```python
from build123d import *

# Parameters (mm, degrees)
SKETCH_1_R      = 4
EXTRUDE_1_DEPTH = 5


with BuildPart() as part:
    # 草图1 → 凸台-拉伸1 (new body)
    with BuildSketch(Plane.XY):
        with BuildLine():
            Line((-7.924938012, 37.574342627), (-22.446516876, 37.574342627))
            Line((-22.446516876, 37.574342627), (-22.446516876, 34.574342627))
            Line((-22.446516876, 34.574342627), (-13.144515754, 34.574342627))
            Line((-13.144515754, 34.574342627), (-13.144515754, 29.574342627))
            Line((-13.144515754, 29.574342627), (-16.675920201, 29.574342627))
            Line((-16.675920201, 29.574342627), (-16.675920201, 3.864736877))
            ThreePointArc((-16.675920201, 3.864736877), (-13.746988013, -3.206330935), (-6.675920201, -6.135263123))
            Line((-6.675920201, -6.135263123), (4.313762442, -6.135263123))
            ThreePointArc((4.313762442, -6.135263123), (7.499853762, 0.046835335), (4.2368016, 6.188659968))
            Line((4.2368016, 6.188659968), (-4.924938012, 6.188659968))
            ThreePointArc((-4.924938012, 6.188659968), (-7.046258356, 7.067339624), (-7.924938012, 9.188659968))
            Line((-7.924938012, 9.188659968), (-7.924938012, 37.574342627))
        make_face()
        Circle(SKETCH_1_R, mode=Mode.SUBTRACT)
    extrude(amount=EXTRUDE_1_DEPTH)


solid = part.part
```
Verification items for the finished model (mm, model axes). A direction names the side the tool comes from. Round coordinates to 2 decimals unless told otherwise and drop trailing zeros. Write each loop counter-clockwise with the first axis right and the second up, starting at its lowest first coordinate (ties: lowest second). Pieces come first, ordered by that corner, then holes. Notation, with made-up numbers: (71, 38) -> (122, 38) arc R31 ccw to (122, 63) -> close; hole circle Ø10 at (61.5, -33). An arc over 180 degrees is marked (long way). Write each question's results on one line, items separated by ' | '.
Q1. Sectioned sample at C-C, the plane y = 0. Record the boundary of the cut face in (x, z).
Derived:
outline: (-15.9, 0) -> (-4, 0) -> (-4, 5) -> (-15.9, 5) -> close; (4, 0) -> (7.5, 0) -> (7.5, 5) -> (4, 5) -> close
Q2. Go/stop test with flat-tipped pins: pin 1 Ø3 at (y, z) = (11.5, 1.5) entering from +X; pin 2 Ø2 at (y, z) = (21.5, 3) entering from -X; pin 3 Ø3 at (x, z) = (-18.5, 1) entering from -Y. Record where each tip stops, or that it passes through.
Derived:
pin 1: stops at x = -7.92 | pin 2: stops at x = -16.68 | pin 3: stops at y = 34.57
Q3. Access from +Z, -Z, +X, -X, +Y, -Y to the whole of each face (thin tool, end or side, straight path). Record for faces 5 (the face through (-15, 29.574, 2)), 6 (the face through (-9, 13, 0)), 7 (the face through (-16.676, 17, 2)), 8 (the face through (-7.925, 23, 2)).
Derived:
face 5: +Z, -Z, -X | face 6: -Z, +X, -X, +Y, -Y | face 7: +Z, -Z, -X, -Y | face 8: +Z, -Z, +X, +Y
Q4. Draft check along Y on faces 1 (the face through (-18, 34.574, 2)), 2 (the face through (-13.145, 32, 2)), 3 (the face through (-9, 13, 5)), 4 (the face through (-1, -6.135, 2)). Enter one of: released by +Y, released by -Y, zero draft, split by the parting line, or undercut.
Derived:
face 1: undercut | face 2: undercut | face 3: zero draft | face 4: released by -Y
Q5. Thickness scan on probe 1 along Y at (x, z) = (0, 2.9); probe 2 along Y at (x, z) = (1.5, 0.65); probe 3 along X at (y, z) = (23, 1.05). Record the ranges inside material, lowest first.
Derived:
probe 1: y = -6.14 to -4, 4 to 6.19 | probe 2: y = -6.14 to -3.71, 3.71 to 6.19 | probe 3: x = -16.68 to -7.92
Q6. Sectioned sample at A-A, the plane z = 1.55. Record the boundary of the cut face in (x, y).
Derived:
outline: (-22.45, 34.57) -> (-13.14, 34.57) -> (-13.14, 29.57) -> (-16.68, 29.57) -> (-16.68, 3.86) arc R10 ccw to (-6.68, -6.14) -> (4.31, -6.14) arc R7.5 ccw to (4.24, 6.19) -> (-4.92, 6.19) arc R3 cw to (-7.92, 9.19) -> (-7.92, 37.57) -> (-22.45, 37.57) -> close; hole circle Ø8 at (0, 0)
Q7. Sectioned sample at B-B, the plane x = 0. Record the boundary of the cut face in (y, z), and give its area (3 significant figures).
Derived:
outline: (-6.14, 0) -> (-4, 0) -> (-4, 5) -> (-6.14, 5) -> close; (4, 0) -> (6.19, 0) -> (6.19, 5) -> (4, 5) -> close | area: 21.6 mm²
Q8. Sectioned sample at D-D, the plane y = 18.5. Record the boundary of the cut face in (x, z), and give its area (3 significant figures).
Derived:
outline: (-16.68, 0) -> (-7.92, 0) -> (-7.92, 5) -> (-16.68, 5) -> close | area: 43.8 mm²
